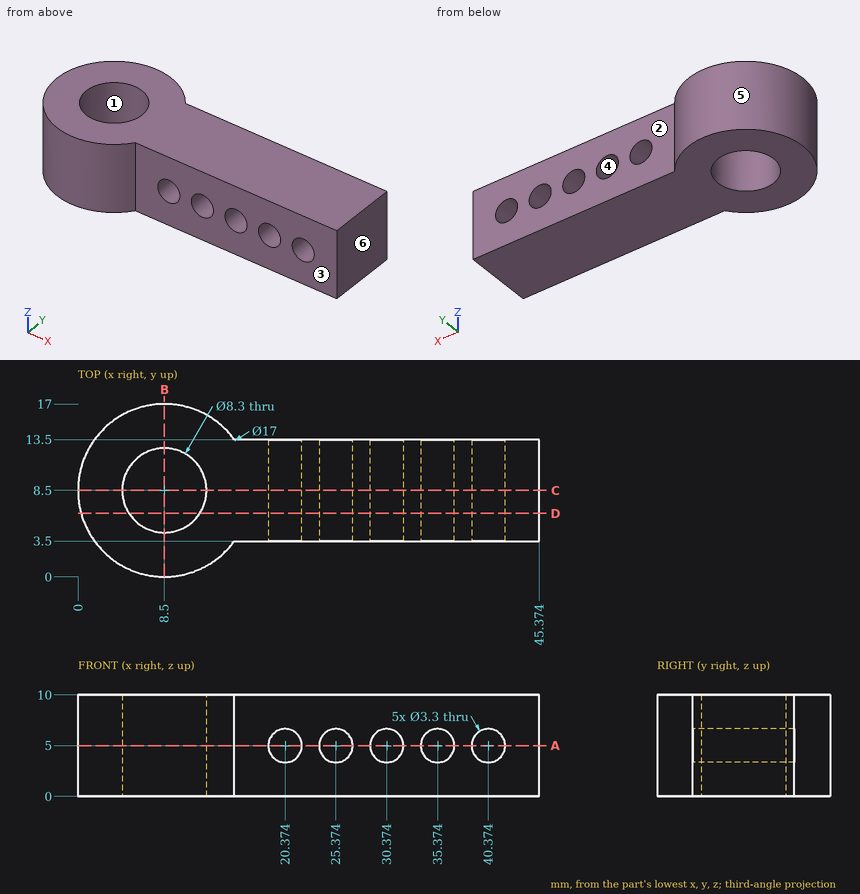
The figure shows three views and two pictorial views of one solid part (mm, origin at its lowest corner). Answer the questions. A direction names the side the tool comes from. Give positions to 0.01 mm unless a question says otherwise; leave off trailing zeros. Order: outer loops, then holes, each group sorted by start corner. A loop starts at its lowest first (then second) coordinate and runs counter-clockwise, first axis right, second up. Notation, with made-up numbers: (53.5, -40) -> (82.5, -40) arc R21 cw to (82.5, -36) -> close; hole circle Ø5 at (-14.75, -8.5). An arc over 180 degrees is marked (long way). Answer as CSV lines item,"result". Start each with the question number.
Q1. A cutting plane is placed at C-C (y = 8.5). Determine the outline of the cut face in (x, z).
Q2. Given pin 1 (2 mm diameter, centred on x = 25.37, z = 5, fed in from -Y); pin 2 (5.5 mm diameter, centred on x = 30.37, z = 5, fed in from -Y); pin 3 (4 mm diameter, centred on x = 19.5, y = 14, fed in from +Z); pin 4 (6 mm diameter, centred on x = 35, z = 5.5, fed in from +Y), each flat-ended and moving along its own axis, determine where each tip first touches the part or whether it passes through.
Q3. A cutting plane is placed at D-D (y = 6.25). Determine the outline of the cut face in (x, z), then the cut area to 3 significant figures.
Q4. Determine the mould class of the marked faces 4, 5 and 6 for opening direction X: pulls with the +X half, pulls with the -X half, needs draft (parallel to the pull), parting line crosses it, or undercut.
Q5. Which of the six approach directions +Z, -Z, +X, -X, +Y, -Y give full straight-line access (tool end or side, diameter ignored) to the marked faces 1, 2 and 3?
Q6. A cutting plane is placed at B-B (x = 8.5). Determine the outline of the cut face in (y, z), then the cut area to 3 significant figures.
Q7. Find the intervals of material crossed by L1, parallel to Y at x = 8.5, z = 8.25; L2, parallel to Y at x = 15.5, z = 9.25; L3, parallel to Y at x = 5, z = 1 (1 decimal), in increasing order.
Q8. A cutting plane is placed at A-A (z = 5). Determine the outline of the cut face in (x, y), then the cut area to 3 significant figures.
Results found:
1,outline,"(0, 0) -> (4.35, 0) -> (4.35, 10) -> (0, 10) -> close; (12.65, 0) -> (45.37, 0) -> (45.37, 10) -> (12.65, 10) -> close; hole circle Ø3.3 at (20.37, 5); hole circle Ø3.3 at (25.37, 5); hole circle Ø3.3 at (30.37, 5); hole circle Ø3.3 at (35.37, 5); hole circle Ø3.3 at (40.37, 5)"
2,pin 1,"through"
2,pin 2,"y = 3.5"
2,pin 3,"z = 10"
2,pin 4,"y = 13.5"
3,outline,"(0.3, 0) -> (5.01, 0) -> (5.01, 10) -> (0.3, 10) -> close; (11.99, 0) -> (45.37, 0) -> (45.37, 10) -> (11.99, 10) -> close; hole circle Ø3.3 at (20.37, 5); hole circle Ø3.3 at (25.37, 5); hole circle Ø3.3 at (30.37, 5); hole circle Ø3.3 at (35.37, 5); hole circle Ø3.3 at (40.37, 5)"
3,area,"338 mm2"
4,face 4,"undercut"
4,face 5,"parting line crosses it"
4,face 6,"pulls with the +X half"
5,face 1,"+Z, -Z"
5,face 2,"+Z, -Z, +X, +Y"
5,face 3,"+Z, -Z, +X, -Y"
6,outline,"(0, 0) -> (4.35, 0) -> (4.35, 10) -> (0, 10) -> close; (12.65, 0) -> (17, 0) -> (17, 10) -> (12.65, 10) -> close"
6,area,"87.0 mm2"
7,L1,"0 to 4.35, 12.65 to 17"
7,L2,"3.5 to 13.5"
7,L3,"0.8 to 6.3, 10.7 to 16.2"
8,outline,"(15.37, 3.5) -> (18.72, 3.5) -> (18.72, 13.5) -> (15.37, 13.5) arc R8.5 ccw (long way) to start; (22.02, 3.5) -> (23.72, 3.5) -> (23.72, 13.5) -> (22.02, 13.5) -> close; (27.02, 3.5) -> (28.72, 3.5) -> (28.72, 13.5) -> (27.02, 13.5) -> close; (32.02, 3.5) -> (33.72, 3.5) -> (33.72, 13.5) -> (32.02, 13.5) -> close; (37.02, 3.5) -> (38.72, 3.5) -> (38.72, 13.5) -> (37.02, 13.5) -> close; (42.02, 3.5) -> (45.37, 3.5) -> (45.37, 13.5) -> (42.02, 13.5) -> close; hole circle Ø8.3 at (8.5, 8.5)"
8,area,"297 mm2"
